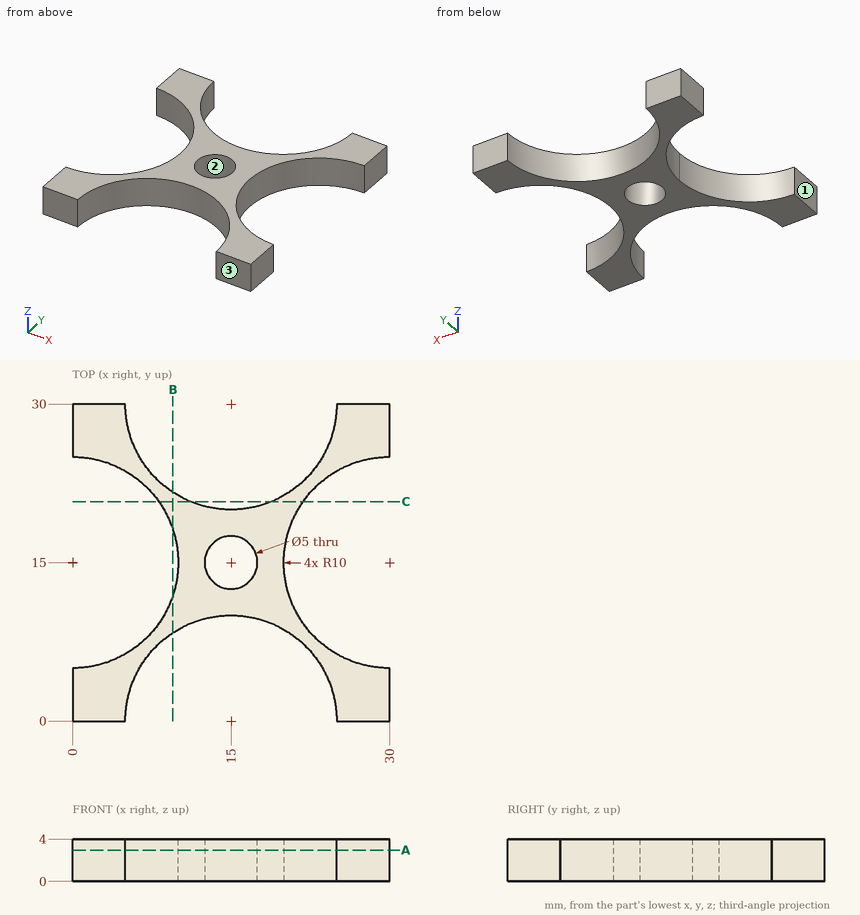
Design review of the part shown in the three views and the two pictorial views. Dimensions are in mm from the part's minimum x, y and z. Give positions to 0.01 mm unless a question says otherwise; leave off trailing zeros. Loops run counter-clockwise (first coordinate to the right, second up) from the corner with the lowest first, then second, coordinate; pieces in that order, holes last. Notation, with made-up numbers: (24, 53.5) -> (71, 53.5) arc R24 cw to (71, 67.5) -> close; hole circle Ø10 at (-33.5, -7.5). An arc over 180 degrees is marked (long way). Answer as a JSON object with one key per item and string values. Group by question number.
Q1. Take a section at A-A (z = 2.95). Write out the cut boundary in (x, y), plus the area to 3 significant figures.
Q2. Wall thickness on line 1 along Y through (x, z) = (15, 1.75); line 2 along Y through (x, z) = (22.25, 3.1); line 3 along X through (y, z) = (12.75, 1.85): over which ranges is each line inside the solid? List them lowest first.
Q3. Draft analysis for pull direction X (two halves, no side actions). For the marked faces 1, 2 and 3, state which applies: pulls with the +X half, pulls with the -X half, needs draft (parallel to the pull), parting line crosses it, or undercut.
Q4. Take a section at B-B (x = 9.5). Write out the cut boundary in (y, z), plus the area to 3 significant figures.
Q5. Take a section at C-C (y = 20.75). Write out the cut boundary in (x, z), plus the area to 3 significant figures.
Answer below:
{
 "1": {"outline": "(0, 0) -> (5, 0) arc R10 cw to (25, 0) -> (30, 0) -> (30, 5) arc R10 cw to (30, 25) -> (30, 30) -> (25, 30) arc R10 cw to (5, 30) -> (0, 30) -> (0, 25) arc R10 cw to (10, 15) arc R10 cw to (0, 5) -> close; hole circle Ø5 at (15, 15)", "area": "252 mm2"},
 "2": {"line 1": "y = 10 to 12.5, 17.5 to 20", "line 2": "y = 6.89 to 8.68, 21.32 to 23.11", "line 3": "x = 9.74 to 13.91, 16.09 to 20.26"},
 "3": {"face 1": "pulls with the -X half", "face 2": "undercut", "face 3": "needs draft"},
 "4": {"outline": "(8.35, 0) -> (11.88, 0) -> (11.88, 4) -> (8.35, 4) -> close; (18.12, 0) -> (21.65, 0) -> (21.65, 4) -> (18.12, 4) -> close", "area": "28.2 mm2"},
 "5": {"outline": "(8.18, 0) -> (11.2, 0) -> (11.2, 4) -> (8.18, 4) -> close; (18.8, 0) -> (21.82, 0) -> (21.82, 4) -> (18.8, 4) -> close", "area": "24.2 mm2"}
}
